The model under review builds one solid part; all positions refer to its coordinate system, in mm. Face numbers are marked on the shaded views. A direction names the side the tool comes from. Round coordinates to 2 decimals unless told otherwise and drop trailing zeros. Order: outer loops, then holes, each group sorted by start corner. A loop starts at its lowest first (then second) coordinate and runs counter-clockwise, first axis right, second up. Notation, with made-up numbers: M 20,72.5 L 27,72.5 A21 cw 27,107.5 Z; hole C 4.5,-12 d10. An arc over 180 degrees is marked long. Answer as a JSON object with one key per item and string values. Group by question number.
1. Add section C-C on z = 26. State the section outline as (x, y) points, and give its area (3 significant figures).
2. Mouldability with a two-part tool opening along Y and no side actions: class the marked faces 3, 4 and 5 as released by +Y, released by -Y, zero draft, split by the parting line, or undercut.
3. Add section B-B on z = 14.75. State the section outline as (x, y) points, and give its area (3 significant figures).
4. Machinability: for the marked faces 1 and 2, which of the approach directions +Z, -Z, +X, -X, +Y, -Y give a long, thin tool a straight path to every point of the face, cutting with its end or side? Answer none if there is none.
5. Add section A-A on y = -15. State the section outline as (x, z) points.
6. To check wall thickness, follow probe 1 along X at (y, z) = (-4, 5.25); probe 2 along Y at (x, z) = (-3.5, 12.5); probe 3 along Z at (x, y) = (10.5, 29.5). State the ranges of each line that lie inside material, in increasing order. Write a range as [from, to].
7. Add section D-D on x = -16. State the section outline as (y, z) points, and give its area (3 significant figures).
8. Clearance check with a flat-ended pin moving along its axis: P1, Ø0.6, axis at x = -36, z = 14, coming from the +Y side. State where the tip first meets the part, or that it passes through.
```python
from build123d import *

# Parameters (mm, degrees)
F1_DEPTH = 5
F3_DEPTH = 25
F4_W     = 10
F4_H     = 12
F4_W_2   = 13
F5_DEPTH = 2.1


with BuildPart() as f1:
    # F0 (on Top) → F1 (new body)
    with BuildSketch(Plane.XY):
        with BuildLine():
            Line((34.28, 32.5), (-34.28, 32.5))
            ThreePointArc((-34.28, 32.5), (-35.694214, 31.914214), (-36.28, 30.5))
            Line((-36.28, 30.5), (-36.28, -30.5))
            ThreePointArc((-36.28, -30.5), (-35.694214, -31.914214), (-34.28, -32.5))
            Line((-34.28, -32.5), (34.28, -32.5))
            ThreePointArc((34.28, -32.5), (35.694214, -31.914214), (36.28, -30.5))
            Line((36.28, -30.5), (36.28, 30.5))
            ThreePointArc((36.28, 30.5), (35.694214, 31.914214), (34.28, 32.5))
        make_face()
    extrude(amount=F1_DEPTH)

    # F2 (on face) → F3 (join)
    with BuildSketch(Plane.XY.offset(5)):
        with BuildLine():
            ThreePointArc((36.28, 30.5), (35.694214, 31.914214), (34.28, 32.5))
            Line((34.28, 32.5), (-34.28, 32.5))
            ThreePointArc((-34.28, 32.5), (-35.694214, 31.914214), (-36.28, 30.5))
            Line((-36.28, 30.5), (-36.28, -30.5))
            ThreePointArc((-36.28, -30.5), (-35.694214, -31.914214), (-34.28, -32.5))
            Line((-34.28, -32.5), (34.28, -32.5))
            ThreePointArc((34.28, -32.5), (35.694214, -31.914214), (36.28, -30.5))
            Line((36.28, -30.5), (36.28, 30.5))
        make_face()
        with BuildLine():
            ThreePointArc((-35.5, 28.5), (-34.914214, 29.914214), (-33.5, 30.5))
            Line((-33.5, 30.5), (33.5, 30.5))
            ThreePointArc((33.5, 30.5), (34.914214, 29.914214), (35.5, 28.5))
            Line((35.5, 28.5), (35.5, -28.5))
            ThreePointArc((35.5, -28.5), (34.914214, -29.914214), (33.5, -30.5))
            Line((33.5, -30.5), (-33.5, -30.5))
            ThreePointArc((-33.5, -30.5), (-34.914214, -29.914214), (-35.5, -28.5))
            Line((-35.5, -28.5), (-35.5, 28.5))
        make_face(mode=Mode.SUBTRACT)
    extrude(amount=F3_DEPTH)

    # F4 (on face) → F5 (cut)
    with BuildSketch(Plane(origin=(-36.28, 0, 0), x_dir=(0, -1, 0), z_dir=(-1, 0, 0))):
        with Locations((16.33, 11)):
            Rectangle(F4_W, F4_H)
        with Locations((-13.57, 11)):
            Rectangle(F4_W_2, F4_H)
    extrude(amount=-F5_DEPTH, mode=Mode.SUBTRACT)


solid = f1.part
```
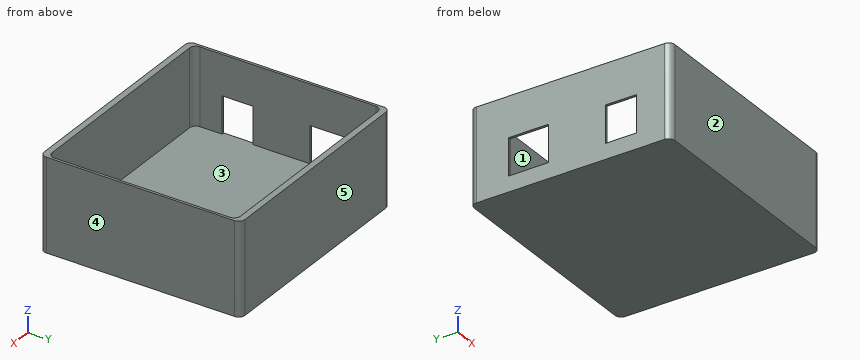
Recorded:
{
 "1": {"outline": "M -36.28,-30.5 A2 ccw -34.28,-32.5 L 34.28,-32.5 A2 ccw 36.28,-30.5 L 36.28,30.5 A2 ccw 34.28,32.5 L -34.28,32.5 A2 ccw -36.28,30.5 Z; hole M -35.5,-28.5 A2 ccw -33.5,-30.5 L 33.5,-30.5 A2 ccw 35.5,-28.5 L 35.5,28.5 A2 ccw 33.5,30.5 L -33.5,30.5 A2 ccw -35.5,28.5 Z", "area": "385 mm²"},
 "2": {"face 3": "undercut", "face 4": "zero draft", "face 5": "released by +Y"},
 "3": {"outline": "M -36.28,-30.5 A2 ccw -34.28,-32.5 L 34.28,-32.5 A2 ccw 36.28,-30.5 L 36.28,30.5 A2 ccw 34.28,32.5 L -34.28,32.5 A2 ccw -36.28,30.5 L -36.28,20.07 L -35.5,20.07 L -35.5,28.5 A2 cw -33.5,30.5 L 33.5,30.5 A2 cw 35.5,28.5 L 35.5,-28.5 A2 cw 33.5,-30.5 L -33.5,-30.5 A2 cw -35.5,-28.5 L -35.5,-21.33 L -36.28,-21.33 Z; M -36.28,-11.33 L -35.5,-11.33 L -35.5,7.07 L -36.28,7.07 Z", "area": "367 mm²"},
 "4": {"face 1": "+Z", "face 2": "+Z, -Z, +X, -X, -Y"},
 "5": {"outline": "M -36.28,0 L 36.28,0 L 36.28,30 L 35.5,30 L 35.5,5 L -36.28,5 Z; M -36.28,17 L -35.5,17 L -35.5,30 L -36.28,30 Z"},
 "6": {"probe 1": "x = [-36.28, -35.5], [35.5, 36.28]", "probe 2": "y = [-32.5, -30.5], [30.5, 32.5]", "probe 3": "z = [0, 5]"},
 "7": {"outline": "M -32.5,0 L 32.5,0 L 32.5,30 L 30.5,30 L 30.5,5 L -30.5,5 L -30.5,30 L -32.5,30 Z", "area": "425 mm²"},
 "8": {"P1": "stops at y = 31.91"}
}
